from build123d import *

# Parameters (mm, degrees)
F1_DEPTH = 5
F2_R     = 2.5
F3_DEPTH = 25
F4_R     = 2.5
F5_DEPTH = 25


with BuildPart() as f1:
    # F0 (on Front) → F1 (new body)
    with BuildSketch(Plane.XZ):
        with BuildLine():
            ThreePointArc((7.071068, 7.071068), (-7.071068, 7.071068), (-7.071068, -7.071068))
            Line((-7.071068, -7.071068), (7.071068, 7.071068))
        make_face()
        Polygon((7.071068, 7.071068), (-7.071068, -7.071068), (192.928932, -207.071068), (207.071068, -192.928932), align=None)
        with BuildLine():
            Line((207.071068, -192.928932), (192.928932, -207.071068))
            ThreePointArc((192.928932, -207.071068), (207.071068, -207.071068), (207.071068, -192.928932))
        make_face()
    extrude(amount=F1_DEPTH)

    # F2 (on face) → F3 (cut)
    with BuildSketch(Plane.XZ.offset(5)):
        Circle(F2_R)
    extrude(amount=-F3_DEPTH, mode=Mode.SUBTRACT)

    # F4 (on face) → F5 (cut)
    with BuildSketch(Plane.XZ.offset(5)):
        with Locations((200, -200)):
            Circle(F4_R)
    extrude(amount=-F5_DEPTH, mode=Mode.SUBTRACT)


solid = f1.part
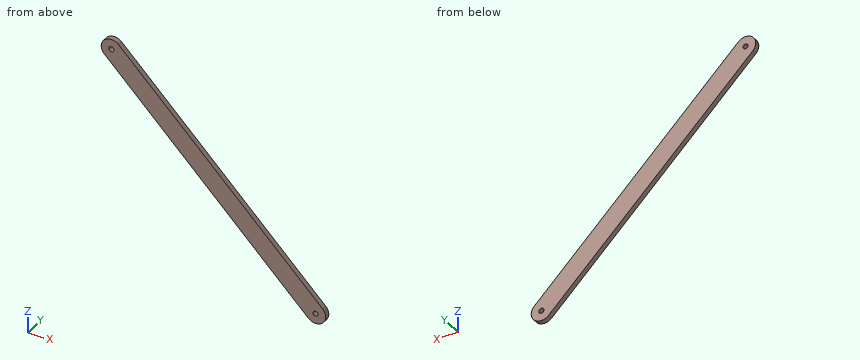
Design review of the part built by this model. Coordinates are the model's own, in mm. Round coordinates to 2 decimals unless told otherwise and drop trailing zeros. Write each loop counter-clockwise with the first axis right and the second up, starting at its lowest first coordinate (ties: lowest second). Pieces come first, ordered by that corner, then holes.
Item 1: Consider section D-D on x = 156.5. Give the boundary of the cut face in (y, z).
Item 2: Consider section A-A on z = -200. Give the boundary of the cut face in (x, y).
Item 3: Consider section B-B on x = 200. Give the boundary of the cut face in (y, z).
Item 4: Consider section C-C on y = -3. Give the boundary of the cut face in (x, z), and give its area (3 significant figures).
Item 5: Wall thickness on L1, parallel to Z at x = 0, y = -2.35; L2, parallel to Z at x = 200, y = -2.2; L3, parallel to X at y = -1.05, z = -200: over which ranges is each line inside the solid? List them lowest first.
Item 6: For pin 1 Ø1 at (y, z) = (-3, -65) entering from -X; pin 2 Ø1 at (x, y) = (32.5, -1) entering from -Z, all flat-tipped, find the tip position at first contact; note any pin that passes through.
Check values:
1. outline: (-5, -170.64) - (0, -170.64) - (0, -142.36) - (-5, -142.36) - close
2. outline: (185.86, -5) - (197.5, -5) - (197.5, 0) - (185.86, 0) - close; (202.5, -5) - (210, -5) - (210, 0) - (202.5, 0) - close
3. outline: (-5, -210) - (0, -210) - (0, -202.5) - (-5, -202.5) - close; (-5, -197.5) - (0, -197.5) - (0, -185.86) - (-5, -185.86) - close
4. outline: (-7.07, -7.07) - (192.93, -207.07) arc R10 ccw to (207.07, -192.93) - (7.07, 7.07) arc R10 ccw to start; hole circle Ø5 at (0, 0); hole circle Ø5 at (200, -200)
4. area: 5,930 mm2
5. L1: z = -14.14 to -2.5, 2.5 to 10
5. L2: z = -210 to -202.5, -197.5 to -185.86
5. L3: x = 185.86 to 197.5, 202.5 to 210
6. pin 1: stops at x = 50.36
6. pin 2: stops at z = -47.14
